Input: part model. Units: mm. Frame: model coordinates. Give positions to 0.01 mm unless a question says otherwise; leave off trailing zeros. Loops run counter-clockwise (first coordinate to the right, second up) from the corner with the lowest first, then second, coordinate; pieces in that order, holes last. Notation, with made-up numbers: (-7, 6) -> (15, 6) arc R25 cw to (15, 43) -> close; hole circle Ø9 at (86.25, -12). An arc over 180 degrees is marked (long way). One line per question, with ' | ' between items.
from build123d import *

# Parameters (mm, degrees)
F0_W     = 304.8
F0_H     = 125.8824
F1_DEPTH = 3.175
F2_W     = 355.6
F2_H     = 177.8
F3_DEPTH = 3.175
F4_DEPTH = 12.7
F5_R     = 25.4
F6_R     = 25.4
F7_R     = 25.4
F8_R     = 25.4


with BuildPart() as f1:
    # F0 (on Top) → F1 (new body, symmetric)
    with BuildSketch(Plane.XY):
        Rectangle(F0_W, F0_H)
    extrude(amount=F1_DEPTH, both=True)

    # F2 (on Top) → F3 (join, symmetric)
    with BuildSketch(Plane.XY):
        Rectangle(F2_W, F2_H)
    extrude(amount=F3_DEPTH, both=True)

    # F0 (on Top) → F4 (cut, symmetric)
    with BuildSketch(Plane.XY):
        Rectangle(F0_W, F0_H)
    extrude(amount=F4_DEPTH, both=True, mode=Mode.SUBTRACT)

    # F5
    f5_edges = [f1.edges().sort_by_distance(p)[0] for p in [
        (-177.8, 88.9, 0),
    ]]
    fillet(f5_edges, radius=F5_R)

    # F6
    f6_edges = [f1.edges().sort_by_distance(p)[0] for p in [
        (177.8, 88.9, 0),
    ]]
    fillet(f6_edges, radius=F6_R)

    # F7
    f7_edges = [f1.edges().sort_by_distance(p)[0] for p in [
        (177.8, -88.9, 0),
    ]]
    fillet(f7_edges, radius=F7_R)

    # F8
    f8_edges = [f1.edges().sort_by_distance(p)[0] for p in [
        (-177.8, -88.9, 0),
    ]]
    fillet(f8_edges, radius=F8_R)


solid = f1.part
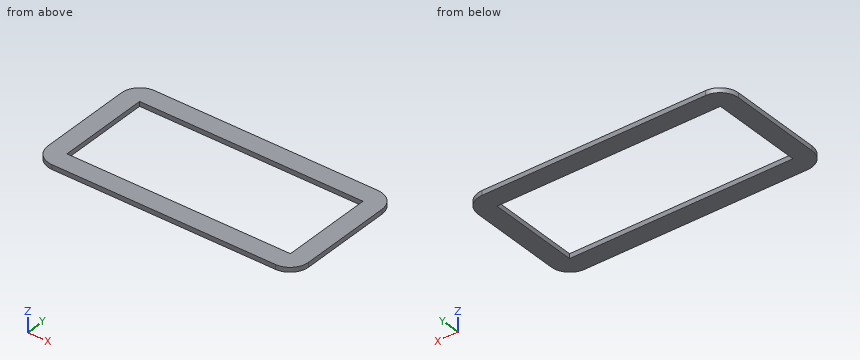
1. Section query A-A (x = 19.5). Output: boundary loops of the cut face in (y, z) (3 decimals).
Determined:
outline: (-88.9, -3.175) -> (-62.941, -3.175) -> (-62.941, 3.175) -> (-88.9, 3.175) -> close; (62.941, -3.175) -> (88.9, -3.175) -> (88.9, 3.175) -> (62.941, 3.175) -> close
2. Section query C-C (z = -1.5). Output: boundary loops of the cut face in (x, y), then the cut area to 3 significant figures.
Determined:
outline: (-177.8, -63.5) arc R25.4 ccw to (-152.4, -88.9) -> (152.4, -88.9) arc R25.4 ccw to (177.8, -63.5) -> (177.8, 63.5) arc R25.4 ccw to (152.4, 88.9) -> (-152.4, 88.9) arc R25.4 ccw to (-177.8, 63.5) -> close; hole (-152.4, -62.94) -> (152.4, -62.94) -> (152.4, 62.94) -> (-152.4, 62.94) -> close | area: 24,300 mm2
3. Pin query (flat end, axial travel): P1, Ø10, axis at x = -0.5, y = -55, coming from the -Z side. Return the tip coordinate at first contact, or that it passes through.
Determined:
P1: passes through
4. Ray query, line 1 along Y through (x, z) = (47, -2.5); line 2 along X through (y, z) = (-42.5, 1.75); line 3 along X through (y, z) = (64, 0.25). Return the intervals inside material, ascending. Write a range as from..to.
Determined:
line 1: y = -88.9..-62.94, 62.94..88.9 | line 2: x = -177.8..-152.4, 152.4..177.8 | line 3: x = -177.8..177.8
5. Section query B-B (y = -45). Output: boundary loops of the cut face in (x, z) (3 decimals), then the cut area to 3 significant figures.
Determined:
outline: (-177.8, -3.175) -> (-152.4, -3.175) -> (-152.4, 3.175) -> (-177.8, 3.175) -> close; (152.4, -3.175) -> (177.8, -3.175) -> (177.8, 3.175) -> (152.4, 3.175) -> close | area: 323 mm2
